Model file for the job. Use its own axes, mm. A direction names the side the tool comes from. Give positions to 0.01 mm unless a question says otherwise; leave off trailing zeros. Loops run counter-clockwise (first coordinate to the right, second up) from the corner with the lowest first, then second, coordinate; pieces in that order, holes last. Notation, with made-up numbers: (62, -15.75) - (66, -15.75) arc R20 cw to (66, -5.75) - close; hole circle Ø5 at (64, -1). An arc over 180 degrees is marked (long way). Answer as CSV lines item,"result". Start each with the question number.
Item 1: Tool access for faces 4 (the flat face through (0, -32, 986)), 5 (the flat face through (0, 35, 986)): list every direction of +Z, -Z, +X, -X, +Y, -Y with a clear straight run to the whole face (end or side of a thin tool).
Item 2: Saw through at C-C on z = 321.5. Give the cut face in (x, y).
Item 3: Pull direction Y, two halves, no side cores. Call faces 1 (the flat face through (0, -35, 986)), 2 (the flat face through (-35, 0, 986)), 3 (the flat face through (32, 0, 986)): pulls with the +Y half, pulls with the -Y half, needs draft (parallel to the pull), parting line crosses it, or undercut.
Item 4: Saw through at A-A on x = -14. Give the cut face in (y, z).
Item 5: Drill centre lines: L1, parallel to Y at x = 30, z = 1168.5; L2, parallel to X at y = 28, z = 863. Where is each one in solid material? Low to high. Write a range as from..to.
Autodesk Inventor part; units mm, degrees
ref_plane "Plano inicial" through (0, 0, -25) normal (0, 0, 1) x (1, 0, 0)
ref_plane "Plano final" through (0, 0, 2025) normal (0, 0, 1) x (1, 0, 0)
ref_plane "YZ Plane" through (0, 0, 0) normal (1, 0, 0) x (0, 1, 0)
ref_plane "Plano inicial" through (0, 0, -25) normal (0, 0, 1) x (1, 0, 0)
ref_plane "Plano final" through (0, 0, 2025) normal (0, 0, 1) x (1, 0, 0)
sketch "Boceto" plane through (0, 0, 0) normal (0, 0, 1) x (1, 0, 0)
  line L0 (-35, -29) -> (-35, 29)
  line L1 (-29, 35) -> (29, 35)
  line L2 (35, 29) -> (35, -29)
  line L3 (29, -35) -> (-29, -35)
  arc A0 (-35, -29) -> (-29, -35) centre (-29, -29) ccw
  arc A1 (35, 29) -> (29, 35) centre (29, 29) ccw
  arc A2 (-29, 35) -> (-35, 29) centre (-29, 29) ccw
  arc A3 (29, -35) -> (35, -29) centre (29, -29) ccw
  arc A4 (-29, 32) -> (-32, 29) centre (-29, 29) ccw
  line L4 (-29, 32) -> (29, 32)
  arc A5 (32, 29) -> (29, 32) centre (29, 29) ccw
  line L5 (32, 29) -> (32, -29)
  arc A6 (29, -32) -> (32, -29) centre (29, -29) ccw
  line L6 (29, -32) -> (-29, -32)
  arc A7 (-32, -29) -> (-29, -32) centre (-29, -29) ccw
  line L7 (-32, -29) -> (-32, 29)
  line L8 (0, 50.7397) -> (0, -50.7397) construction
  line L9 (-50.7397, 0) -> (50.7397, 0) construction
  dimension "d7" = 6
  dimension "d9" = 70
  dimension "d11" = 70
  dimension "d12" = 3
  dimension "d15" = 35
  dimension "d16" = 35
extrude "Cuerpo" add sketch "Boceto" along normal up to surface (2050 mm away) from surface at -25
sketch "Sketch3" plane through (0, 0, 0) normal (0, 0, 1) x (1, 0, 0)
  line L0 (0, 0) -> (10, 0)
ref_plane "Work Plane3" through (0, 0, 0) normal (0, -1, 0) x (1, 0, 0)
sketch "Sketch4" plane through (0, 0, 0) normal (0, -1, 0) x (1, 0, 0)
  line L0 (-2, -25) -> (12, -25)
  line L1 (-2, 2025) -> (12, 2025)
  dimension "d18" = 2050
equation "\"d7\" = G_IR"
equation "\"d9\" = G_W"
equation "\"d11\" = G_H"
equation "\"d12\" = G_T"
equation "\"d15\" = 0.5 * d9"
equation "\"d16\" = 0.5 * d11"
equation "\"d3\" = G_L"
equation "\"G_W\" = 70"
equation "\"G_H\" = 70"
equation "\"G_T\" = 3"
equation "\"G_IR\" = 6"
equation "\"G_L\" = d18"
equation "\"G_OFFSET_START\" = 25"
equation "\"G_OFFSET_END\" = 25"
equation "\"d13\" = -G_OFFSET_START"
equation "\"d14\" = G_OFFSET_END + B_L"
properties part number "ISO 10799-2 - 70x70x3 - 2050" material "Galvanizado catalogo 2"
Responses:
1,face 4,"+Z, -Z"
1,face 5,"+Z, -Z, +X, -X, +Y"
2,outline,"(-35, -29) arc R6 ccw to (-29, -35) - (29, -35) arc R6 ccw to (35, -29) - (35, 29) arc R6 ccw to (29, 35) - (-29, 35) arc R6 ccw to (-35, 29) - close; hole (-32, -29) arc R3 ccw to (-29, -32) - (29, -32) arc R3 ccw to (32, -29) - (32, 29) arc R3 ccw to (29, 32) - (-29, 32) arc R3 ccw to (-32, 29) - close"
3,face 1,"pulls with the -Y half"
3,face 2,"needs draft"
3,face 3,"undercut"
4,outline,"(-35, -25) - (-32, -25) - (-32, 2025) - (-35, 2025) - close; (32, -25) - (35, -25) - (35, 2025) - (32, 2025) - close"
5,L1,"-34.92..-31.83, 31.83..34.92"
5,L2,"-35..-32, 32..35"
